```python
from build123d import *

# Parameters (mm, degrees)
PAD_DEPTH = 10


with BuildPart() as part:
    # Sketch → Pad (new body)
    with BuildSketch(Plane.XY):
        with BuildLine():
            Line((66.675, -198.640068), (66.675, 0))
            ThreePointArc((66.675, 0), (49.1691, 45.032823), (5.843948, 66.4184))
            Line((6.259361, 44.007078), (5.843948, 66.4184))
            ThreePointArc((0, -44.45), (44.339131, -3.137506), (6.259361, 44.007078))
            ThreePointArc((-14, -42.187706), (-7.090803, -43.880782), (0, -44.45))
            Line((-14, -198.640068), (-14, -42.187706))
            Line((0, -198.640068), (-14, -198.640068))
            Line((0, -198.640068), (66.675, -198.640068))
        make_face()
    extrude(amount=PAD_DEPTH)


solid = part.part
```
Model file for the job. Use its own axes, mm. Give positions to 0.01 mm unless a question says otherwise; leave off trailing zeros. Order: outer loops, then holes, each group sorted by start corner. A loop starts at its lowest first (then second) coordinate and runs counter-clockwise, first axis right, second up.
1) Saw through at D-D, the plane y = -9. Write the cut outline in (x, z) (3 decimals), then the cut area to 3 significant figures.
2) Saw through at A-A, the plane z = 4.75. Write the cut outline in (x, y) (3 decimals), then the cut area to 3 significant figures.
3) Saw through at C-C, the plane x = 48. Write the cut outline in (y, z), then the cut area to 3 significant figures.
4) Wall check: probe 1 along Y at (x, z) = (14, 3.75); probe 2 along Y at (x, z) = (10.5, 9.5); probe 3 along Y at (x, z) = (-1, 8.5). Give the ranges that are in metal, low to high.
5) Mould opens along X. For faces 1 (the flat face through (-14, -122, 5)), 2 (the flat face through (26, -94, 0)), 3 (the flat face through (66.675, -101, 5)) say: +X half, -X half, draft (parallel to the pull), parting line (faces both ways), or undercut.
6) Pin check, flat tips, straight feed: pin 1 (1.5 mm diameter, centred on y = 33.5, z = 2.5, fed in from +X); pin 2 (5 mm diameter, centred on y = 16.5, z = 3.5, fed in from -X); pin 3 (2 mm diameter, centred on y = -38, z = 8.5, fed in from -X). Stop position of each tip, or through.
7) Saw through at B-B, the plane x = 35. Write the cut outline in (y, z).
Computed:
1. outline: (43.529, 0) - (66.675, 0) - (66.675, 10) - (43.529, 10) - close
1. area: 231 mm2
2. outline: (-14, -198.64) - (66.675, -198.64) - (66.675, 0) arc R66.675 ccw to (5.844, 66.418) - (6.259, 44.007) arc R44.45 cw to (0, -44.45) arc R44.45 cw to (-14, -42.188) - close
2. area: 15,700 mm2
3. outline: (-198.64, 0) - (46.28, 0) - (46.28, 10) - (-198.64, 10) - close
3. area: 2,450 mm2
4. probe 1: y = -198.64 to -42.19, 42.19 to 65.19
4. probe 2: y = -198.64 to -43.19, 43.19 to 65.84
4. probe 3: y = -198.64 to -44.44
5. face 1: -X half
5. face 2: draft
5. face 3: +X half
6. pin 1: stops at x = 58.08
6. pin 2: stops at x = 40.18
6. pin 3: stops at x = 21.33
7. outline: (-198.64, 0) - (-27.4, 0) - (-27.4, 10) - (-198.64, 10) - close; (27.4, 0) - (56.75, 0) - (56.75, 10) - (27.4, 10) - close
